Answer from the drawing. Dimensions are ordinates in mm from the lowest x, y and z of the part. A direction names the side the tool comes from. Round coordinates to 2 decimals unless told otherwise and drop trailing zeros. Write each loop counter-clockwise with the first axis right and the second up, starting at its lowest first coordinate (ties: lowest second). Pieces come first, ordered by that corner, then holes. Notation, with made-up numbers: (73.25, 6.25) - (104.25, 6.25) arc R17 ccw to (104.25, 31.25) - close; hole circle Ø7 at (15, 68). An arc over 180 degrees is marked (long way). Use a Markdown table: item, result. Add a question column.
1) Each of these flat-tipped pins is pushed along its axis until it touches: P1, Ø12, axis at x = 22.5, y = 19, coming from the +Z side; P2, Ø10, axis at x = 48, z = 19.5, coming from the +Y side; P3, Ø2.5, axis at y = 11.5, z = 16.5, coming from the -X side; P4, Ø4, axis at x = 48, z = 11.5, coming from the -Y side. Where does it stop, or does it pass through?
2) A cutting plane is placed at D-D (x = 6). Give the vertices of the cut face in (y, z).
3) Determine the mould class of the marked faces 5, 6 and 7 for opening direction Z: +Z half, -Z half, draft (parallel to the pull), parting line (faces both ways), or undercut.
4) A cutting plane is placed at A-A (z = 8). Give the vertices of the cut face in (x, y).
5) A tool of negligible diameter and unlimited length cuts with its end or side. For the marked faces 1, 2, 3 and 4, from which of +Z, -Z, +X, -X, +Y, -Y can it reach the whole face along a straight path? Write none if from no direction.
6) A cutting plane is placed at B-B (z = 28). Give the vertices of the cut face in (x, y), then the cut area to 3 significant figures.
7) Find the intervals of material crossed by probe 1 along Z at (x, y) = (8.5, 12.5); probe 2 along Z at (x, y) = (27, 10.25); probe 3 along Z at (x, y) = (39, 18.25), in increasing order. Write a range as from..to.
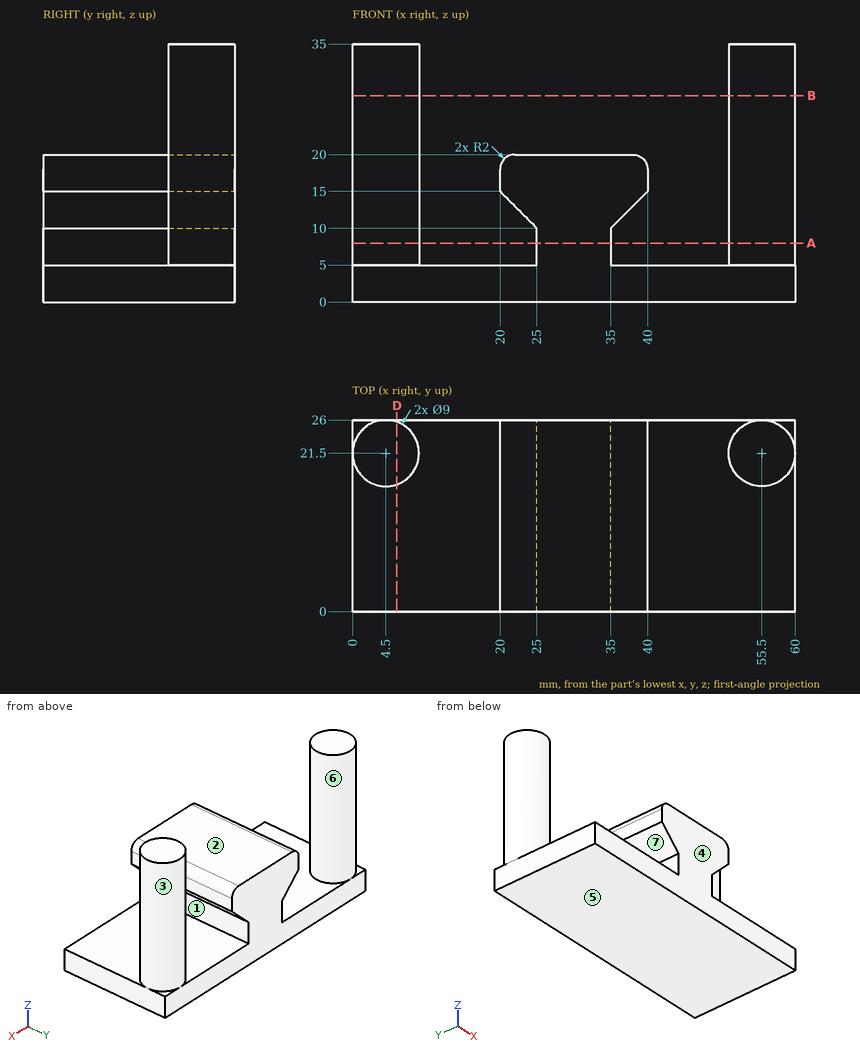
Entries:
| question | item | result |
|---|---|---|
| 1 | P1 | stops at z = 20 |
| 1 | P2 | stops at y = 25.24 |
| 1 | P3 | stops at x = 20 |
| 1 | P4 | passes through |
| 2 | outline | (0, 0) - (26, 0) - (26, 5) - (25.74, 5) - (25.74, 35) - (17.26, 35) - (17.26, 5) - (0, 5) - close |
| 3 | face 5 | -Z half |
| 3 | face 6 | draft |
| 3 | face 7 | undercut |
| 4 | outline | circle Ø9 at (4.5, 21.5); (25, 0) - (35, 0) - (35, 26) - (25, 26) - close; circle Ø9 at (55.5, 21.5) |
| 5 | face 1 | +Y, -Y |
| 5 | face 2 | +Z, +Y, -Y |
| 5 | face 3 | +Z |
| 5 | face 4 | +Z, -Z, +X, -X, -Y |
| 6 | outline | circle Ø9 at (4.5, 21.5); circle Ø9 at (55.5, 21.5) |
| 6 | area | 127 mm² |
| 7 | probe 1 | z = 0..5 |
| 7 | probe 2 | z = 0..20 |
| 7 | probe 3 | z = 0..5, 14..19.73 |
